Autodesk Inventor part; units mm, degrees
ref_plane "YZ Plane" through (0, 0, 0) normal (1, 0, 0) x (0, 1, 0)
ref_plane "XZ Plane" through (0, 0, 0) normal (0, 1, 0) x (-1, 0, 0)
ref_plane "XY Plane" through (0, 0, 0) normal (0, 0, 1) x (1, 0, 0)
sketch "Sketch1" plane through (0, 0, 0) normal (1, 0, 0) x (0, 1, 0)
  line L0 (0, 0) -> (15.875, 0)
  line L1 (15.875, 0) -> (15.875, -25.4)
  line L2 (0, -25.4) -> (0, 0)
  line L3 (4.7625, -25.4) -> (5.9323, -25.4)
  line L4 (4.7625, -25.4) -> (4.7625, -4.7625)
  line L5 (4.7625, -4.7625) -> (11.1125, -4.7625)
  line L6 (11.1125, -4.7625) -> (11.1125, -25.4)
  line L7 (15.875, -25.4) -> (11.1125, -25.4)
  line L8 (4.7625, -25.4) -> (0, -25.4)
  dimension "d1" = 25.4
  dimension "d4" = 6.35
  dimension "d6" = 4.7625
  dimension "d15" = 25.4
  dimension "d22" = 4.7625
  dimension "d24" = 4.7625
extrude "Extrusion1" add sketch "Sketch1" along normal blind 12.7
fillet "Fillet2" radius 0.381 22 edges at (12.7, 15.875, -12.7) (12.7, 11.1125, -15.0813) (0, 15.875, -12.7) (12.7, 7.9375, 0) (12.7, 7.9375, -4.7625) (12.7, 4.7625, -15.0812) (12.7, 0, -12.7) (12.7, 13.4938, -25.4) (12.7, 2.3813, -25.4) (6.35, 15.875, 0) (0, 7.9375, 0) (6.35, 0, 0) (6.35, 15.875, -25.4) (6.35, 4.7625, -25.4) (0, 11.1125, -15.0813) (0, 7.9375, -4.7625) (0, 4.7625, -15.0812) (6.35, 11.1125, -25.4) (0, 13.4938, -25.4) (0, 2.3813, -25.4) (0, 0, -12.7) (6.35, 0, -25.4)
sketch "Sketch6" plane through (0.381, 0.381, 0) normal (0, 0, 1) x (1, 0, 0)
  line L0 (0, 0) -> (0, 15.113)
  line L1 (11.938, 0) -> (0, 0)
  line L2 (11.938, 15.113) -> (11.938, 0)
  line L3 (0, 15.113) -> (11.938, 15.113)
  point P0 (-0.381, -0.381)
  point P1 (6.1556, 7.3722)
hole "Hole1" at (6.5366, 7.7532, 0) direction (0, 0, -1) diameter 3.81 end through all
sketch "Sketch7" plane through (0.381, 0.381, 0) normal (0, 0, 1) x (1, 0, 0)
  circle A0 centre (6.1556, 7.3722) radius 1.905
  line L0 (0, 0) -> (0, 15.113)
  line L1 (11.938, 0) -> (0, 0)
  line L2 (11.938, 15.113) -> (11.938, 0)
  line L3 (0, 15.113) -> (11.938, 15.113)
  point P0 (-0.381, -0.381)
hole "Hole2" at (6.5366, 7.7532, 0) direction (0, 0, -1) diameter 9.525 depth 3.175 tip angle 118
equation "\"d15\" = d1"
properties part number "TensionerAxleHolder"
For this review, take the finished solid that the model builds, in its own axes (mm). A direction names the side the tool comes from. Coordinates: 2 decimals unless noted, no trailing zeros. Loops run counter-clockwise (first coordinate to the right, second up) from the corner with the lowest first, then second, coordinate; pieces in that order, holes last. Notation, with made-up numbers: (9.5, 38) - (50.5, 38) arc R18 ccw to (50.5, 43) - close; hole circle Ø7 at (-6.75, 36.5). An arc over 180 degrees is marked (long way). Return JSON: item names as keys, results as strings.
Item 1: Mouldability with a two-part tool opening along X and no side actions: class faces 3 (the cylindrical face through (5.11, 3.21, -1.61)), 4 (the flat face through (6, 15.875, -13)), 5 (the flat face through (12.7, 3, -10)), 6 (the flat face through (0, 3, -10)) as pulls with the +X half, pulls with the -X half, needs draft (parallel to the pull), parting line crosses it, or undercut.
Determined:
{"face 3": "undercut", "face 4": "needs draft", "face 5": "pulls with the +X half", "face 6": "pulls with the -X half"}
Item 2: Insertion check: pin 1 (1 mm diameter, centred on x = 9, y = 2.5, fed in from +Z); pin 2 (3 mm diameter, centred on x = 5.5, y = 7.5, fed in from -Z); pin 3 (5.5 mm diameter, centred on x = 6.54, y = 7.75, fed in from +Z). Each pin has a flat end and moves straight along its axis. Give the tip position at first contact, or say it passes through.
Determined:
{"pin 1": "stops at z = 0", "pin 2": "stops at z = -4.76", "pin 3": "stops at z = -4.38"}
Item 3: For faces 1 (the flat face through (6, 11.112, -15)), 2 (the flat face through (6, 2, -25.4)), list the 3-axis set-ups (+Z, -Z, +X, -X, +Y, -Y) from which the entire face can be reached by the end or side of a thin tool; tool diameter is ignored.
Determined:
{"face 1": "-Z, +X, -X", "face 2": "-Z, +X, -X, +Y, -Y"}
Item 4: Take a section at A-A (z = -8.25). Give the boundary of the cut face in (x, y) (1 decimal).
Determined:
{"outline": "(0, 0.4) arc R0.4 ccw to (0.4, 0) - (12.3, 0) arc R0.4 ccw to (12.7, 0.4) - (12.7, 4.4) arc R0.4 ccw to (12.3, 4.8) - (0.4, 4.8) arc R0.4 ccw to (0, 4.4) - close; (0, 11.5) arc R0.4 ccw to (0.4, 11.1) - (12.3, 11.1) arc R0.4 ccw to (12.7, 11.5) - (12.7, 15.5) arc R0.4 ccw to (12.3, 15.9) - (0.4, 15.9) arc R0.4 ccw to (0, 15.5) - close"}
Item 5: For line 1 (Y direction, x = 5.5, z = -18.5) (1 decimal); line 2 (X direction, y = 6.75, z = -2.5); line 3 (Z direction, x = 4.5, y = 11.5), list the stretches that pass through material, from the lowest coordinate up.
Determined:
{"line 1": "y = 0 to 4.8, 11.1 to 15.9", "line 2": "x = 0 to 1.88, 11.19 to 12.7", "line 3": "z = -25.4 to -3.47"}
